Build history of the part. All positions in model axes, mm. Face numbers are marked on the shaded views. A direction names the side the tool comes from. Give positions to 0.01 mm unless a question says otherwise; leave off trailing zeros. Write each loop counter-clockwise with the first axis right and the second up, starting at its lowest first coordinate (ties: lowest second). Pieces come first, ordered by that corner, then holes. Notation, with made-up numbers: M 41,-36.5 L 88,-36.5 A18 cw 88,-8.5 Z; hole C 19.25,-35.75 d7. An arc over 180 degrees is marked long. Return JSON: item names as keys, results as strings. Group by question number.
Q1. Band-saw the part on B-B, the plane y = 7.5. Give the cut face in (x, z), then the cut area to 3 significant figures.
Q2. Flat gauge pins, fed straight in: pin 1 Ø10 at (x, z) = (-6.5, 1) entering from +Y; pin 2 Ø4 at (y, z) = (1.5, 2.5) entering from -X; pin 3 Ø0.7 at (x, y) = (0, 1.5) entering from +Z; pin 4 Ø1.5 at (y, z) = (1.5, 9.5) entering from -X. Where does each tip first touch, or does it go through?
Q3. Tool access for the marked faces 4, 5 and 6: list every direction of +Z, -Z, +X, -X, +Y, -Y with a clear straight run to the whole face (end or side of a thin tool).
Q4. Band-saw the part on A-A, the plane x = 0. Give the cut face in (y, z).
Q5. Pull direction Z, two halves, no side cores. Call the marked faces 1, 2 and 3: +Z half, -Z half, draft (parallel to the pull), parting line (faces both ways), or undercut.
Q6. Wall check: probe 1 along X at (y, z) = (8, 0); probe 2 along Y at (x, z) = (10, -1.25); probe 3 along X at (y, z) = (6.75, 0). Give the ranges that are in metal, low to high.
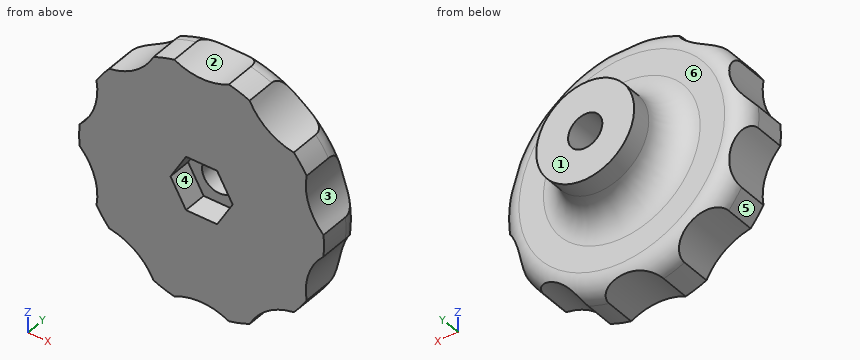
from build123d import *

# Parameters (mm, degrees)
FILETE1_R             = 3
FILETE2_R             = 2
ESBO_O2_R             = 6
CORTE_EXTRUS_O1_DEPTH = 5
PADR_OCIRCULAR1_COUNT = 10
ESBO_O3_R             = 1.75
CORTE_EXTRUS_O2_DEPTH = 10
CORTE_EXTRUS_O3_DEPTH = 2.4


with BuildPart() as part:
    # Esboço1 → Revolução1 (revolve)
    with BuildSketch(Plane.XY, mode=Mode.PRIVATE) as revolu_o1_sk:
        Polygon((0, 0), (12.5, 0), (12.5, 5), (5, 5), (5, 10), (0, 10), align=None)
    revolve(revolu_o1_sk.sketch.rotate(Axis((0, 0, 0), (0, 1, 0)), 90), axis=Axis((0, 0, 0), (0, 1, 0)))

    # Filete1
    filete1_edges = [part.edges().sort_by_distance(p)[0] for p in [
        (0, 5, 5),
    ]]
    fillet(filete1_edges, radius=FILETE1_R)

    # Filete2
    filete2_edges = [part.edges().sort_by_distance(p)[0] for p in [
        (0, 5, 12.5),
    ]]
    fillet(filete2_edges, radius=FILETE2_R)

    # Esboço2 → Corte-extrusão1 (cut)
    with BuildSketch(Plane.XZ):
        with Locations((0, 17.5)):
            Circle(ESBO_O2_R)
    corte_extrus_o1 = extrude(amount=-CORTE_EXTRUS_O1_DEPTH, mode=Mode.SUBTRACT)

    # PadrãoCircular1: Corte-extrusão1 ×10 about axis
    padr_ocircular1_axis = Axis((0, 0, 0), (0, 1, 0))
    for i in range(1, PADR_OCIRCULAR1_COUNT):
        add(corte_extrus_o1.rotate(padr_ocircular1_axis, i * 360 / PADR_OCIRCULAR1_COUNT), mode=Mode.SUBTRACT)

    # Esboço3 → Corte-extrusão2 (cut)
    with BuildSketch(Plane.XZ):
        with Locations(Location((0, 0, 0), (0, 0, 270))):
            Circle(ESBO_O3_R)
    extrude(amount=-CORTE_EXTRUS_O2_DEPTH, mode=Mode.SUBTRACT)

    # Esboço4 → Corte-extrusão3 (cut)
    with BuildSketch(Plane.XZ):
        Polygon((3.175426481, 0), (1.58771324, 2.75), (-1.58771324, 2.75), (-3.175426481, 0), (-1.58771324, -2.75), (1.58771324, -2.75), align=None)
    extrude(amount=-CORTE_EXTRUS_O3_DEPTH, mode=Mode.SUBTRACT)


solid = part.part
From the geometry:
{
 "1": {"outline": "C 0,0 d10.08; hole C 0,0 d3.5", "area": "70.2 mm^2"},
 "2": {"pin 1": "stops at y = 10", "pin 2": "stops at x = -12.49", "pin 3": "stops at z = 11.51", "pin 4": "stops at x = -7.69"},
 "3": {"face 4": "-Y", "face 5": "-Z, -X, +Y, -Y", "face 6": "+Y"},
 "4": {"outline": "M 0,-11.5 L 4.73,-11.5 A2 ccw 5,-10.5 L 5,-8 A3 cw 8,-5 L 10,-5 L 10,-1.75 L 2.4,-1.75 L 2.4,-2.75 L 0,-2.75 Z; M 0,2.75 L 2.4,2.75 L 2.4,1.75 L 10,1.75 L 10,5 L 8,5 A3 cw 5,8 L 5,10.5 A2 ccw 4.73,11.5 L 0,11.5 Z"},
 "5": {"face 1": "draft", "face 2": "+Z half", "face 3": "undercut"},
 "6": {"probe 1": "x = -5 to -1.75, 1.75 to 5", "probe 2": "y = 0 to 5", "probe 3": "x = -5.27 to -1.75, 1.75 to 5.27"}
}
